Could you check a few things on this model? Use its own coordinates, in mm. A direction names the side the tool comes from. Round coordinates to 2 decimals unless told otherwise and drop trailing zeros. One line per question, with ' | ' between items.
```python
from build123d import *

# Parameters (mm, degrees)
BOSS_EXTRUDE1_OUTLINE_R   = 2.5
BOSS_EXTRUDE1_OUTLINE_R_2 = 4.7
BOSS_EXTRUDE1_OUTLINE_R_3 = 5.8
BOSS_EXTRUDE1_OUTLINE_R_4 = 2
BOSS_EXTRUDE1_DEPTH       = 3
SKETCH3_R                 = 1.5
CUT_EXTRUDE1_DEPTH        = 2
SKETCH4_R                 = 6.65
CUT_EXTRUDE3_DEPTH        = 1


# Read off the part's stored shape, not the designer's step: Boss-Extrude1
with BuildPart() as part:
    # Boss-Extrude1 outline → Boss-Extrude1 (new body)
    with BuildSketch(Plane(origin=(0, 0, 0), x_dir=(1, 0, 0), z_dir=(0, 1, 0))):
        with BuildLine():
            Line((-70, 78), (-119.123426788, 72.331912294))
            add(Edge.make_bspline(
                [(-119.123426788, 72.331912294), (-121.817313074, 72.000000019), (-122.273896674, 69.717527721)],
                knots=[0.016356922, 0.016356922, 0.016356922, 0.873306336, 0.873306336, 0.873306336], degree=2))
            Line((-122.273896674, 69.717527721), (-125, 47))
            add(Edge.make_bspline(
                [(-125, 47), (-140.310843166, 12.049240253), (-122.843906966, -52.183993971)],
                knots=[0, 0, 0, 0.96415889, 0.96415889, 0.96415889], degree=2))
            add(Edge.make_bspline(
                [(-122.843906966, -52.183993971), (-121.5, -57), (-118.282004102, -60.826813609)],
                knots=[0, 0, 0, 1, 1, 1], degree=2))
            add(Edge.make_bspline(
                [(-118.282004102, -60.826813609), (-103.606996493, -76.952025301), (-86.5, -72)],
                knots=[0.099631764, 0.099631764, 0.099631764, 1, 1, 1], degree=2))
            add(Edge.make_bspline(
                [(-86.5, -72), (0, -60), (86.5, -72)],
                knots=[0, 0, 0, 1, 1, 1], degree=2, weights=[1, 1.666666667, 1]))
            add(Edge.make_bspline(
                [(118.282004106, -60.826813605), (103.606996495, -76.952025301), (86.5, -72)],
                knots=[0.099631763, 0.099631763, 0.099631763, 1, 1, 1], degree=2))
            add(Edge.make_bspline(
                [(122.843906966, -52.183993971), (121.5, -57), (118.282004106, -60.826813605)],
                knots=[0, 0, 0, 1, 1, 1], degree=2))
            add(Edge.make_bspline(
                [(125, 47), (140.310843171, 12.049240242), (122.843906966, -52.183993971)],
                knots=[0, 0, 0, 0.96415889, 0.96415889, 0.96415889], degree=2))
            Line((125, 47), (122.273896674, 69.717527721))
            add(Edge.make_bspline(
                [(119.123426788, 72.331912294), (121.817313074, 72.000000019), (122.273896674, 69.717527721)],
                knots=[0.016356922, 0.016356922, 0.016356922, 0.873306336, 0.873306336, 0.873306336], degree=2))
            Line((119.123426788, 72.331912294), (70, 78))
            add(Edge.make_bspline(
                [(-70, 78), (0, 81), (70, 78)],
                knots=[0, 0, 0, 1, 1, 1], degree=2, weights=[1, 1.857142857, 1]))
        make_face()
        with Locations((-101.086868344, -59.874042945)):
            Circle(BOSS_EXTRUDE1_OUTLINE_R, mode=Mode.SUBTRACT)
        with Locations((-32.460031949, -46.153127094)):
            Circle(BOSS_EXTRUDE1_OUTLINE_R_2, mode=Mode.SUBTRACT)
        with Locations((-117.25, -21)):
            Circle(BOSS_EXTRUDE1_OUTLINE_R, mode=Mode.SUBTRACT)
        with BuildLine():
            Line((-70, -12), (-70, -29))
            add(Edge.make_bspline(
                [(-70, -29), (-70, -31.999987298), (-71.652526625, -34.50382822)],
                knots=[0, 0, 0, 1, 1, 1], degree=2))
            Line((-71.652526625, -34.50382822), (-85.673736688, -55.74808589))
            add(Edge.make_bspline(
                [(-85, -3), (-99, -3), (-112, 0), (-108, -8.5), (-105, -31), (-98, -49), (-94.5, -57), (-86.500030089, -57), (-85.673736688, -55.74808589)],
                knots=[0, 0, 0, 0, 0, 0, 0, 0, 0, 1, 1, 1, 1, 1, 1, 1, 1, 1], degree=8))
            Line((-85, -3), (-79, -3))
            ThreePointArc((-79, -3), (-72.636038969, -5.636038969), (-70, -12))
        make_face(mode=Mode.SUBTRACT)
        with Locations((-57.5, -23.153127094)):
            Circle(BOSS_EXTRUDE1_OUTLINE_R_3, mode=Mode.SUBTRACT)
        with Locations((0, -27.5)):
            Circle(BOSS_EXTRUDE1_OUTLINE_R_4, mode=Mode.SUBTRACT)
        with Locations((-23.815698604, -13.75)):
            Circle(BOSS_EXTRUDE1_OUTLINE_R_4, mode=Mode.SUBTRACT)
        with Locations((32.460031949, -46.153127094)):
            Circle(BOSS_EXTRUDE1_OUTLINE_R_2, mode=Mode.SUBTRACT)
        with Locations((101.086868344, -59.874042945)):
            Circle(BOSS_EXTRUDE1_OUTLINE_R, mode=Mode.SUBTRACT)
        with Locations((57.5, -23.153127094)):
            Circle(BOSS_EXTRUDE1_OUTLINE_R_3, mode=Mode.SUBTRACT)
        with Locations((23.815698604, -13.75)):
            Circle(BOSS_EXTRUDE1_OUTLINE_R_4, mode=Mode.SUBTRACT)
        with BuildLine():
            add(Edge.make_bspline(
                [(85, -3), (99, -3), (112, 0), (108, -8.5), (105, -31), (98, -49), (94.5, -57), (86.500030089, -57), (85.673736688, -55.74808589)],
                knots=[0, 0, 0, 0, 0, 0, 0, 0, 0, 1, 1, 1, 1, 1, 1, 1, 1, 1], degree=8))
            Line((85.673736688, -55.74808589), (71.652526625, -34.50382822))
            add(Edge.make_bspline(
                [(70, -29), (70, -31.999987298), (71.652526625, -34.50382822)],
                knots=[0, 0, 0, 1, 1, 1], degree=2))
            Line((70, -29), (70, -12))
            ThreePointArc((70, -12), (72.636038969, -5.636038969), (79, -3))
            Line((79, -3), (85, -3))
        make_face(mode=Mode.SUBTRACT)
        with Locations((117.25, -21)):
            Circle(BOSS_EXTRUDE1_OUTLINE_R, mode=Mode.SUBTRACT)
        with Locations((-88, 6)):
            Circle(BOSS_EXTRUDE1_OUTLINE_R, mode=Mode.SUBTRACT)
        with Locations((-117.3, 34.5)):
            Circle(BOSS_EXTRUDE1_OUTLINE_R, mode=Mode.SUBTRACT)
        with BuildLine():
            add(Edge.make_bspline(
                [(-105, 42), (-108, 15), (-92, 15), (-83.5, 15)],
                knots=[0, 0, 0, 0, 1, 1, 1, 1], degree=3))
            add(Edge.make_bspline(
                [(-85, 51), (-102.75, 51), (-105, 42)],
                knots=[0, 0, 0, 1, 1, 1], degree=2))
            ThreePointArc((-85, 51), (-74.393398282, 46.606601718), (-70, 36))
            Line((-70, 36), (-70, 24))
            ThreePointArc((-70, 24), (-72.636038969, 17.636038969), (-79, 15))
            Line((-79, 15), (-83.5, 15))
        make_face(mode=Mode.SUBTRACT)
        with Locations((-64.577794898, 6)):
            Circle(BOSS_EXTRUDE1_OUTLINE_R_3, mode=Mode.SUBTRACT)
        with Locations((-23.815698604, 13.75)):
            Circle(BOSS_EXTRUDE1_OUTLINE_R_4, mode=Mode.SUBTRACT)
        with Locations((-57.5, 29.977172881)):
            Circle(BOSS_EXTRUDE1_OUTLINE_R_3, mode=Mode.SUBTRACT)
        with Locations((0, 27.5)):
            Circle(BOSS_EXTRUDE1_OUTLINE_R_4, mode=Mode.SUBTRACT)
        with Locations((-111, 58)):
            Circle(BOSS_EXTRUDE1_OUTLINE_R_3, mode=Mode.SUBTRACT)
        with Locations((-86.612529585, 63.500116978)):
            Circle(BOSS_EXTRUDE1_OUTLINE_R_3, mode=Mode.SUBTRACT)
        with Locations((-63.376133298, 54.276783114)):
            Circle(BOSS_EXTRUDE1_OUTLINE_R_3, mode=Mode.SUBTRACT)
        with Locations((-31, 55.5)):
            Circle(BOSS_EXTRUDE1_OUTLINE_R_4, mode=Mode.SUBTRACT)
        with Locations((-31, 73.5)):
            Circle(BOSS_EXTRUDE1_OUTLINE_R_4, mode=Mode.SUBTRACT)
        with Locations((23.815698604, 13.75)):
            Circle(BOSS_EXTRUDE1_OUTLINE_R_4, mode=Mode.SUBTRACT)
        with Locations((64.577794898, 6)):
            Circle(BOSS_EXTRUDE1_OUTLINE_R_3, mode=Mode.SUBTRACT)
        with Locations((57.5, 29.977172881)):
            Circle(BOSS_EXTRUDE1_OUTLINE_R_3, mode=Mode.SUBTRACT)
        with Locations((88, 6)):
            Circle(BOSS_EXTRUDE1_OUTLINE_R, mode=Mode.SUBTRACT)
        with BuildLine():
            ThreePointArc((70, 36), (74.393398282, 46.606601718), (85, 51))
            add(Edge.make_bspline(
                [(85, 51), (102.75, 51), (105, 42)],
                knots=[0, 0, 0, 1, 1, 1], degree=2))
            add(Edge.make_bspline(
                [(105, 42), (108, 15), (92, 15), (83.5, 15)],
                knots=[0, 0, 0, 0, 1, 1, 1, 1], degree=3))
            Line((83.5, 15), (79, 15))
            ThreePointArc((79, 15), (72.636038969, 17.636038969), (70, 24))
            Line((70, 24), (70, 36))
        make_face(mode=Mode.SUBTRACT)
        with Locations((117.3, 34.5)):
            Circle(BOSS_EXTRUDE1_OUTLINE_R, mode=Mode.SUBTRACT)
        with Locations((31, 55.5)):
            Circle(BOSS_EXTRUDE1_OUTLINE_R_4, mode=Mode.SUBTRACT)
        with Locations((63.376133298, 54.276783114)):
            Circle(BOSS_EXTRUDE1_OUTLINE_R_3, mode=Mode.SUBTRACT)
        with Locations((31, 73.5)):
            Circle(BOSS_EXTRUDE1_OUTLINE_R_4, mode=Mode.SUBTRACT)
        with Locations((111, 58)):
            Circle(BOSS_EXTRUDE1_OUTLINE_R_3, mode=Mode.SUBTRACT)
        with Locations((86.612529585, 63.500116978)):
            Circle(BOSS_EXTRUDE1_OUTLINE_R_3, mode=Mode.SUBTRACT)
    extrude(amount=BOSS_EXTRUDE1_DEPTH)

    # Sketch3 → Cut-Extrude1 (cut)
    with BuildSketch(Plane.XZ):
        with Locations(Location((-25.085243816, 42.803127094, 0), (0, 0, 270))):
            Circle(SKETCH3_R)
        with Locations(Location((39.834820081, 42.803127094, 0), (0, 0, 270))):
            Circle(SKETCH3_R)
    extrude(amount=-CUT_EXTRUDE1_DEPTH, mode=Mode.SUBTRACT)

    # Sketch4 → Cut-Extrude3 (cut)
    with BuildSketch(Plane(origin=(0, 3, 0), x_dir=(1, 0, 0), z_dir=(0, 1, 0))):
        with Locations(Location((-57.5, 29.977172881, 0), (0, 0, 270))):
            Circle(SKETCH4_R)
        with Locations(Location((-63.376133298, 54.276783114, 0), (0, 0, 270))):
            Circle(SKETCH4_R)
        with Locations(Location((-86.612529585, 63.500116978, 0), (0, 0, 270))):
            Circle(SKETCH4_R)
        with Locations(Location((-111, 58, 0), (0, 0, 270))):
            Circle(SKETCH4_R)
        with Locations(Location((-64.577794898, 6, 0), (0, 0, 270))):
            Circle(SKETCH4_R)
        with Locations(Location((-57.5, -23.153127094, 0), (0, 0, 270))):
            Circle(SKETCH4_R)
        with Locations(Location((57.5, -23.153127094, 0), (0, 0, 90))):
            Circle(SKETCH4_R)
        with Locations(Location((64.577794898, 6, 0), (0, 0, 90))):
            Circle(SKETCH4_R)
        with Locations(Location((111, 58, 0), (0, 0, 90))):
            Circle(SKETCH4_R)
        with Locations(Location((86.612529585, 63.500116978, 0), (0, 0, 90))):
            Circle(SKETCH4_R)
        with Locations(Location((63.376133298, 54.276783114, 0), (0, 0, 90))):
            Circle(SKETCH4_R)
        with Locations(Location((57.5, 29.977172881, 0), (0, 0, 90))):
            Circle(SKETCH4_R)
    extrude(amount=-CUT_EXTRUDE3_DEPTH, mode=Mode.SUBTRACT)


solid = part.part
```
1. I'm going to push flat-ended pins straight in: pin 1 (10.5 mm diameter, centred on x = -108.5, z = -56.5, fed in from +Y); pin 2 (10.5 mm diameter, centred on x = -64.58, z = -6, fed in from +Y). Where does each tip first touch, or does it pass through?
From the geometry:
pin 1: stops at y = 3 | pin 2: passes through
2. If we mould it in two halves opening along X, with no side actions, what happens to faces 1 (the face through (94.906, 1.479, -75.126)), 2 (the face through (74.28, 1.48, -46.49)), 3 (the face through (-94.218, 1.479, -75.206))? For each: pulls with the +X half, pulls with the -X half, needs draft (parallel to the pull), parting line crosses it, or undercut.
From the geometry:
face 1: pulls with the +X half | face 2: undercut | face 3: pulls with the -X half
3. On a 3-axis mill with a long thin cutter (end or side, diameter ignored), from which of +Z, -Z, +X, -X, +Y, -Y can I reach the whole of each face in a straight line? I mean faces 4 (the face through (70.477, 2.507, -9.069)), 5 (the face through (78.76, 1.48, 45.27)). Say none if no direction works.
From the geometry:
face 4: +Y | face 5: +Y, -Y
4. I need wall thicknesses on probe 1 along X at (y, z) = (1, -31); probe 2 along Z at (x, y) = (84.5, 1); probe 3 along X at (y, z) = (1.9, -40). Which ranges of each line are inside material? Lowest first, please.
From the geometry:
probe 1: x = -129.99 to -105.09, -70 to -63.21, -51.79 to 51.79, 63.21 to 70, 105.09 to 129.99 | probe 2: z = -76.33 to -68.9, -58.1 to -50.99, -15 to 3, 53.97 to 71.72 | probe 3: x = -127.64 to -105.19, -70.54 to 70.54, 105.19 to 127.64
5. I want a section at A-A on y = 1.35. Count the separate pieces of the cut face and the enclosed holes in it, and give its area (3 significant figures).
From the geometry:
separate pieces: 1 | enclosed holes: 38 | area: 30,200 mm²
